from build123d import *

# Parameters (mm, degrees)
SKETCH1_R           = 3.15
BOSS_EXTRUDE1_DEPTH = 3
SKETCH2_R           = 5
BOSS_EXTRUDE2_DEPTH = 3
FILLET1_R           = 1
CUT_EXTRUDE1_REACH  = 11.274
SKETCH3_R           = 1.65
SKETCH4_R           = 3
CUT_EXTRUDE2_DEPTH  = 2.5


with BuildPart() as part:
    # Sketch1 → Boss-Extrude1 (new body)
    with BuildSketch(Plane.XY):
        Circle(SKETCH1_R)
    extrude(amount=BOSS_EXTRUDE1_DEPTH)

    # Sketch2 → Boss-Extrude2 (add)
    with BuildSketch(Plane(origin=(0, 0, 0), x_dir=(-1, 0, 0), z_dir=(0, 0, -1))):
        Circle(SKETCH2_R)
    extrude(amount=BOSS_EXTRUDE2_DEPTH)

    # Fillet1
    fillet1_edges = [part.edges().sort_by_distance(p)[0] for p in [
        (-3.15, 0, 0),
    ]]
    fillet(fillet1_edges, radius=FILLET1_R)

    # Sketch3 → Cut-Extrude1 (cut, up to next)
    with BuildSketch(Plane(origin=(0, 0, -3), x_dir=(-1, 0, 0), z_dir=(0, 0, -1)), mode=Mode.PRIVATE) as cut_extrude1_sk1:
        Circle(SKETCH3_R)
    cut_extrude1_tool1 = extrude(cut_extrude1_sk1.sketch, amount=-CUT_EXTRUDE1_REACH, mode=Mode.PRIVATE) & part.part
    add(cut_extrude1_tool1.solids().sort_by_distance((0, 0, -3))[0], mode=Mode.SUBTRACT)

    # Sketch4 → Cut-Extrude2 (cut)
    with BuildSketch(Plane(origin=(0, 0, -3), x_dir=(-1, 0, 0), z_dir=(0, 0, -1))):
        Circle(SKETCH4_R)
    extrude(amount=-CUT_EXTRUDE2_DEPTH, mode=Mode.SUBTRACT)


solid = part.part
Read the model definition and answer for the solid it produces. Units are mm, in the model's axes. A direction names the side the tool comes from. Coordinates: 2 decimals unless noted, no trailing zeros. Loops run counter-clockwise (first coordinate to the right, second up) from the corner with the lowest first, then second, coordinate; pieces in that order, holes last.
Q1. Consider probe 1 along Y at (x, z) = (0, -1.75); probe 2 along Y at (x, z) = (0, 2.4); probe 3 along Z at (x, y) = (-1, -2.25). Determine where each line is inside the solid, lowest interval first.
Q2. The mould has two halves that part along X. Classify faces 4 (the face through (1.4, -1.4, 3)), 5 (the face through (-2.5, -1.917, 1.986)), 6 (the face through (1.216, 1.115, 1.226)): +X half, -X half, draft (parallel to the pull), parting line (faces both ways), or undercut.
Q3. Which of the six approach directions +Z, -Z, +X, -X, +Y, -Y give full straight-line access (tool end or side, diameter ignored) to faces 1 (the face through (0.1, -3.3, -3)), 2 (the face through (-1.3, -1.3, -0.5)), 3 (the face through (2, 4, 0))?
Q4. The part is cut by section C-C on z = -1.75. Write down the section's boundary in (x, y), and give its area (3 significant figures).
Q5. The part is cut by section A-A on y = 0. Write down the section's boundary in (x, z), and give its area (3 significant figures).
Q6. The part is cut by section D-D on z = 1.75. Write down the section's boundary in (x, y).
Q7. Each of these flat-tipped pins is pushed along its axis until it touches: pin 1 Ø2 at (y, z) = (3, -1) entering from +X; pin 2 Ø3 at (x, y) = (-1, 0.5) entering from -Z. Where does it stop, or does it pass through?
Results below:
1. probe 1: y = -5 to -3, 3 to 5
1. probe 2: y = -3.15 to -1.65, 1.65 to 3.15
1. probe 3: z = -0.5 to 3
2. face 4: draft
2. face 5: parting line
2. face 6: undercut
3. face 1: -Z, +X, -X, +Y, -Y
3. face 2: -Z
3. face 3: +Z
4. outline: circle Ø10 at (0, 0); hole circle Ø6 at (0, 0)
4. area: 50.3 mm2
5. outline: (-5, -3) - (-3, -3) - (-3, -0.5) - (-1.65, -0.5) - (-1.65, 3) - (-3.15, 3) - (-3.15, 1) arc R1 cw to (-4.15, 0) - (-5, 0) - close; (1.65, -0.5) - (3, -0.5) - (3, -3) - (5, -3) - (5, 0) - (4.15, 0) arc R1 cw to (3.15, 1) - (3.15, 3) - (1.65, 3) - close
5. area: 22.8 mm2
6. outline: circle Ø6.3 at (0, 0); hole circle Ø3.3 at (0, 0)
7. pin 1: stops at x = 4.58
7. pin 2: stops at z = -0.5
